Here's the drawing with two shaded views (mm, measured from the low corner). I have some questions. Give positions to 0.01 mm unless a question says otherwise; leave off trailing zeros. Loops run counter-clockwise (first coordinate to the right, second up) from the corner with the lowest first, then second, coordinate; pieces in that order, holes last. Notation, with made-up numbers: M 8,-14 L 54,-14 A30 cw 54,21 Z; hole C 47.5,18.25 d6. An arc over 180 degrees is marked long. Put each result on its own line as item: value. Start each with the question number.
1) For P1, Ø1, axis at y = 18, z = 23.5, coming from the -X side; P2, Ø1.5, axis at x = 30.5, z = 18, coming from the -Y side; P3, Ø2, axis at x = 36, y = 31.5, coming from the -Z side; P4, Ø10, axis at x = 9.5, z = 10.5, coming from the -Y side (1 decimal), each with a flat end and sliding along its axis, tell me the tip position at first contact or that it passes through.
2) Imagine slicing it at D-D (y = 3.5). Write out the boundary of the cut face in (x, z).
3) If we mould it in two halves opening along X, with no side actions, what happens to the marked faces 1, 2, 3 and 4? For each: +X half, -X half, draft (parallel to the pull), parting line (faces both ways), or undercut.
4) Imagine slicing it at A-A (x = 20). Write out the boundary of the cut face in (y, z).
5) Please list where these lines run through material, in increasing order: line 1 along Y through (x, z) = (28.5, 18) (1 decimal); line 2 along Z through (x, y) = (19, 17); line 3 along Y through (x, z) = (20, 15.25). Write a range as from..to.
6) Imagine slicing it at B-B (z = 18.75). Write out the boundary of the cut face in (x, y).
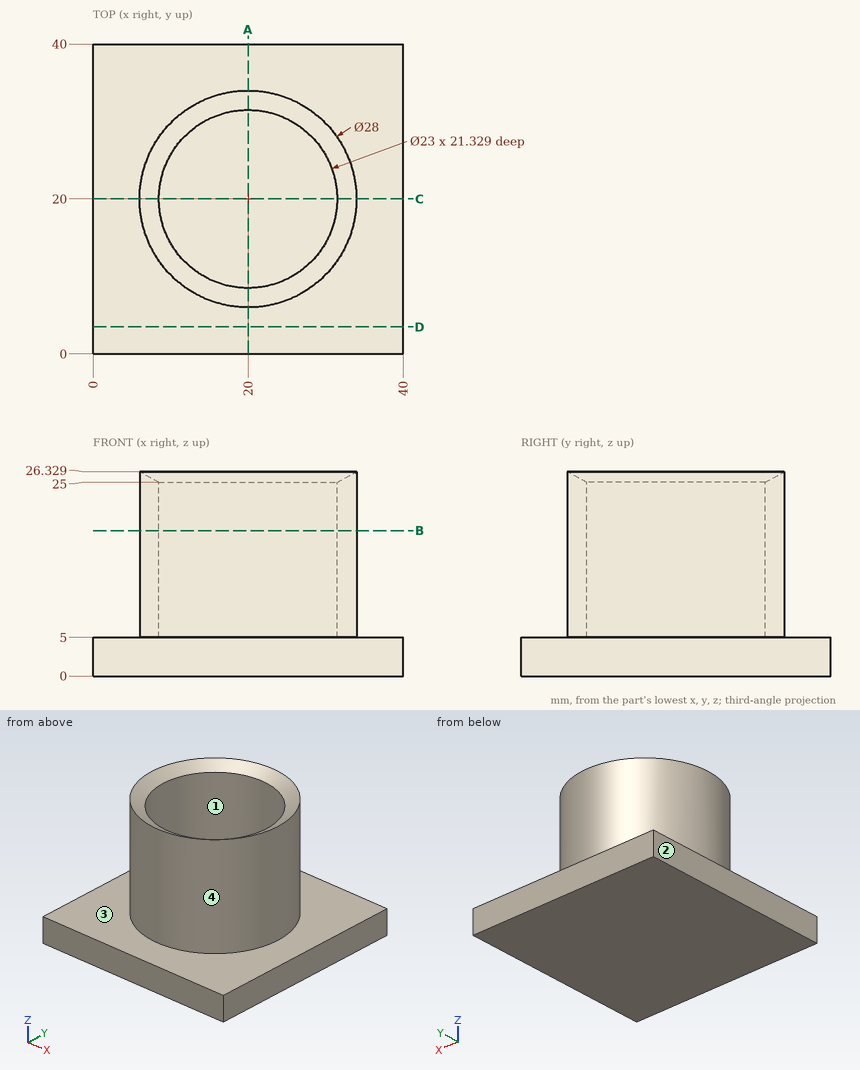
Recorded:
1. P1: x = 6.08
1. P2: y = 9.95
1. P3: z = 0
1. P4: y = 7.1
2. outline: M 0,0 L 40,0 L 40,5 L 0,5 Z
3. face 1: undercut
3. face 2: -X half
3. face 3: draft
3. face 4: parting line
4. outline: M 0,0 L 40,0 L 40,5 L 34,5 L 34,26.33 L 31.5,25 L 31.5,5 L 8.5,5 L 8.5,25 L 6,26.33 L 6,5 L 0,5 Z
5. line 1: 8.9..12.3, 27.7..31.1
5. line 2: 0..5
5. line 3: 6..8.5, 31.5..34
6. outline: C 20,20 d28; hole C 20,20 d23
